from build123d import *

# Parameters (mm, degrees)
F1_R          = 1.905
F2_DEPTH      = 82.55
F2_DEPTH_BACK = 57.15
F3_DEPTH      = 0.762


with BuildPart() as f2:
    # F1 (on Right) → F2 (new body, two sides)
    with BuildSketch(Plane.YZ) as f2_sk:
        Circle(F1_R)
    extrude(amount=F2_DEPTH)
    extrude(f2_sk.sketch, amount=-F2_DEPTH_BACK)

    # F1 (on Right) → F3 (join)
    with BuildSketch(Plane.YZ):
        Circle(F1_R)
    extrude(amount=F3_DEPTH)

    # F0 (on Top) → F4 (revolve)
    with BuildSketch(Plane.XY):
        Polygon((-7.007087, 24.25808), (-16.030946, 24.25808), (-32.2088, 11.899154), (-36.560226, 12.075871), (-39.70601, 4.431527), (-39.70601, 0), (-35.594656, 0), (59.655344, 0), (59.655344, 4.410799), (56.168538, 11.90574), (51.813526, 11.90574), (35.630643, 24.25808), (26.606784, 24.25808), (26.606784, 29.221201), (22.094855, 29.221201), (22.094855, 49.07369), (19.599697, 49.07369), (19.599697, 29.221201), (0, 29.221201), (0, 49.07369), (-2.495158, 49.07369), (-2.495158, 29.221201), (-7.007087, 29.221201), align=None)
    revolve(axis=Axis((0, 0, 0), (-1, 0, 0)))


solid = f2.part
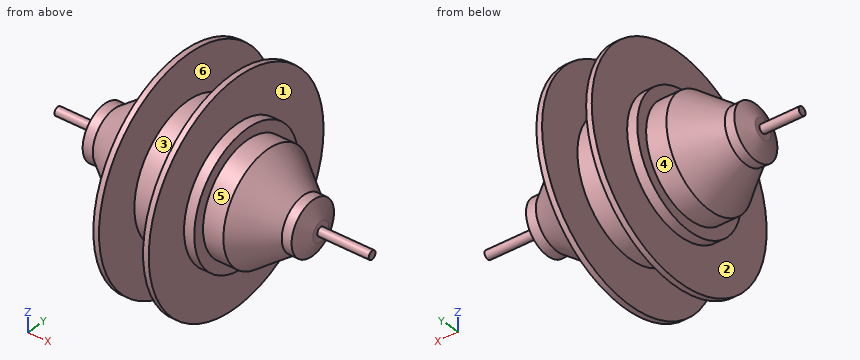
Input: part model. Units: mm. Frame: model coordinates. Face numbers are marked on the shaded views. A direction names the side the tool comes from. Round coordinates to 2 decimals unless told otherwise and drop trailing zeros. Write each loop counter-clockwise with the first axis right and the second up, starting at its lowest first coordinate (ties: lowest second). Pieces come first, ordered by that corner, then holes.
1) Cut plane A-A (z = -38.5). Return the cut outline in (x, y).
2) Contact query for flat-ended pins moving along their axis: P1, Ø3, axis at x = -29.5, z = 5.5, coming from the -Y side; P2, Ø8, axis at x = -31.5, z = 6.5, coming from the -Y side; P3, Ø5, axis at y = -15, z = 2.5, coming from the -X side. Output: stop coordinate, or through.
3) Draft query along X for the marked faces 1, 2 and 3. Return one class per face: pulls with the +X half, pulls with the -X half, needs draft (parallel to the pull), parting line crosses it, or undercut.
4) Cut plane C-C (x = 54). Return the cut outline in (y, z), then the cut area to 3 significant figures.
5) Ray query, L1, parallel to X at y = 31.5, z = -16; L2, parallel to Z at x = -15.5, y = 1; L3, parallel to Z at x = -30, y = -8. Return the intervals inside material, ascending.
6) Cut plane B-B (y = 41.5). Return the cut outline in (x, z), then the cut area to 3 significant figures.
7) Reachability of the marked faces 4, 5 and 6 from +Z, -Z, +X, -X, +Y, -Y: full face, straight path, thin tool, end or side. Return the list, or none.
Geometry says:
1. outline: (-2.5, -30.43) - (0, -30.43) - (0, 30.43) - (-2.5, 30.43) - close; (19.6, -30.43) - (22.09, -30.43) - (22.09, 30.43) - (19.6, 30.43) - close
2. P1: stops at y = -14.2
2. P2: stops at y = -14.43
2. P3: stops at x = -31.15
3. face 1: pulls with the +X half
3. face 2: pulls with the -X half
3. face 3: undercut
4. outline: circle Ø23.81 at (0, 0)
4. area: 445 mm2
5. L1: x = -2.5 to 0, 19.6 to 22.09
5. L2: z = -24.24 to 24.24
5. L3: z = -10.98 to 10.98
6. outline: (-2.5, -26.19) - (0, -26.19) - (0, 26.19) - (-2.5, 26.19) - close; (19.6, -26.19) - (22.09, -26.19) - (22.09, 26.19) - (19.6, 26.19) - close
6. area: 261 mm2
7. face 4: -X
7. face 5: +X
7. face 6: none
